Read the model definition and answer for the solid it produces. Units are mm, in the model's axes. A direction names the side the tool comes from. Coordinates: 2 decimals unless noted, no trailing zeros. Order: outer loops, then holes, each group sorted by start corner. A loop starts at its lowest first (then second) coordinate and runs counter-clockwise, first axis right, second up. Notation, with made-up numbers: M 2.5,-23 L 11.5,-23 A25 ccw 11.5,-8 Z; hole C 62.5,-11 d6. An arc over 180 degrees is marked long. Use a Markdown table: item, result. Add a question column.
1) Find section D-D on x = 4.5. Write down the section's boundary in (y, z), plus the area to 3 significant figures.
2) For faces 5 (the face through (0, 23.812, 25)), 6 (the face through (12.7, -11, 14)), determine the directions among +Z, -Z, +X, -X, +Y, -Y from which every point of the face is accessible in a straight line to the end or side of a thin tool.
3) This flat-tipped pin is pushed along its axis until it touches: pin 1 Ø17 at (y, z) = (0, 25.4) entering from -X. Where does it stop, or does it pass through?
4) Find the intervals of material crossed by probe 1 along X at (y, z) = (-22, 33); probe 2 along Y at (x, z) = (-6, 22); probe 3 along Y at (x, z) = (-12.1, 25.4), in increasing order. Write a range as [from, to].
5) Find section A-A on y = -20.5. Write down the section's boundary in (x, z).
6) The mould has two halves that part along Y. Classify faces 1 (the face through (0, -25.4, 25)), 2 (the face through (-10.635, 23.36, 25.044)), 3 (the face through (11.3, 2, 0)), 4 (the face through (11.895, 0.628, 11.126)): released by +Y, released by -Y, zero draft, split by the parting line, or undercut.
7) Find section C-C on y = 0. Write down the section's boundary in (x, z), plus the area to 3 significant figures.
from build123d import *

# Parameters (mm, degrees)
BOSS_EXTRUDE1_DEPTH = 50.8
SKETCH2_R           = 14.2875
CUT_EXTRUDE1_DEPTH  = 50.8


with BuildPart() as part:
    # Sketch1 → Boss-Extrude1 (new body)
    with BuildSketch(Plane(origin=(0, 0, 0), x_dir=(-1, 0, 0), z_dir=(0, 0, -1))):
        with BuildLine():
            Line((-12.7, 25.146), (-12.7, -25.146))
            ThreePointArc((-12.7, -25.146), (-12.625605122, -25.325605122), (-12.446, -25.4))
            Line((-12.446, -25.4), (12.446, -25.4))
            ThreePointArc((12.446, -25.4), (12.625605122, -25.325605122), (12.7, -25.146))
            Line((12.7, -25.146), (12.7, 25.146))
            ThreePointArc((12.7, 25.146), (12.625605122, 25.325605122), (12.446, 25.4))
            Line((12.446, 25.4), (-12.446, 25.4))
            ThreePointArc((-12.446, 25.4), (-12.625605122, 25.325605122), (-12.7, 25.146))
        make_face()
        with BuildLine():
            Line((-11.1125, -22.225), (-11.1125, 22.225))
            ThreePointArc((-11.1125, 22.225), (-10.647532015, 23.347532015), (-9.525, 23.8125))
            Line((-9.525, 23.8125), (9.525, 23.8125))
            ThreePointArc((9.525, 23.8125), (10.647532015, 23.347532015), (11.1125, 22.225))
            Line((11.1125, 22.225), (11.1125, -22.225))
            ThreePointArc((11.1125, -22.225), (10.647532015, -23.347532015), (9.525, -23.8125))
            Line((9.525, -23.8125), (-9.525, -23.8125))
            ThreePointArc((-9.525, -23.8125), (-10.647532015, -23.347532015), (-11.1125, -22.225))
        make_face(mode=Mode.SUBTRACT)
    extrude(amount=-BOSS_EXTRUDE1_DEPTH)

    # Sketch2 → Cut-Extrude1 (cut)
    with BuildSketch(Plane.ZY.offset(12.7)):
        with Locations((25.4, 0)):
            Circle(SKETCH2_R)
    extrude(amount=-CUT_EXTRUDE1_DEPTH, mode=Mode.SUBTRACT)


solid = part.part
Check result:
| question | item | result |
|---|---|---|
| 1 | outline | M -25.4,0 L -23.81,0 L -23.81,50.8 L -25.4,50.8 Z; M 23.81,0 L 25.4,0 L 25.4,50.8 L 23.81,50.8 Z |
| 1 | area | 161 mm2 |
| 2 | face 5 | +Z, -Z |
| 2 | face 6 | +Z, -Z, +X, +Y, -Y |
| 3 | pin 1 | passes through |
| 4 | probe 1 | x = [-12.7, -11.11], [11.11, 12.7] |
| 4 | probe 2 | y = [-25.4, -23.81], [23.81, 25.4] |
| 4 | probe 3 | y = [-25.4, -14.29], [14.29, 25.4] |
| 5 | outline | M -12.7,0 L -11.11,0 L -11.11,50.8 L -12.7,50.8 Z; M 11.11,0 L 12.7,0 L 12.7,50.8 L 11.11,50.8 Z |
| 6 | face 1 | released by -Y |
| 6 | face 2 | undercut |
| 6 | face 3 | zero draft |
| 6 | face 4 | undercut |
| 7 | outline | M -12.7,0 L -11.11,0 L -11.11,11.11 L -12.7,11.11 Z; M -12.7,39.69 L -11.11,39.69 L -11.11,50.8 L -12.7,50.8 Z; M 11.11,0 L 12.7,0 L 12.7,11.11 L 11.11,11.11 Z; M 11.11,39.69 L 12.7,39.69 L 12.7,50.8 L 11.11,50.8 Z |
| 7 | area | 70.6 mm2 |
